Can you work these out from the model? Positions are in its coordinate system, mm. A direction names the side the tool comes from. Round coordinates to 2 decimals unless told otherwise and drop trailing zeros. One line per item, written item: value. Start each with the question number.
(1) I'm going to push flat-ended pins straight in: pin 1 Ø1.5 at (x, z) = (20, 6) entering from +Y; pin 2 Ø1 at (x, z) = (-0.5, 9.5) entering from +Y. Where does each tip first touch, or does it pass through?
(2) If I drill on L1, parallel to X at y = 33, z = 9.25; L2, parallel to X at y = 141.75, z = 6; L3, parallel to Z at x = 20, y = 140, over which ranges is the centre line in solid material (lowest first)? Write a range as from..to.
(3) Thinking about a two-plate mould opening in X: for faces 3 (the face through (72.5, -2, 5)), 4 (the face through (-1, 2, 0)), 5 (the face through (-42.44, 83.61, 9.68)), which applies, +X half, -X half, draft (parallel to the pull), parting line (faces both ways), or undercut?
(4) On a 3-axis mill with a long thin cutter (end or side, diameter ignored), from which of +Z, -Z, +X, -X, +Y, -Y can I reach the whole of each face in a straight line? I mean faces 1 (the face through (1, 145, 5)), 2 (the face through (43.94, 83.625, 9.679)). Say none if no direction works.
Autodesk Inventor part; units mm, degrees
ref_plane "YZ Plane" through (0, 0, 0) normal (1, 0, 0) x (0, 1, 0)
ref_plane "XZ Plane" through (0, 0, 0) normal (0, 1, 0) x (-1, 0, 0)
ref_plane "XY Plane" through (0, 0, 0) normal (0, 0, 1) x (1, 0, 0)
sketch "Sketch1" plane through (0, 0, 0) normal (0, 0, 1) x (1, 0, 0)
  line L0 (-72.5, -145) -> (72.5, -145)
  line L1 (72.5, -145) -> (72.5, 145)
  line L2 (72.5, 145) -> (-72.5, 145)
  line L3 (-72.5, 145) -> (-72.5, -145)
  line L4 (-72.5, -145) -> (72.5, 145) construction
  line L5 (72.5, -145) -> (-72.5, 145) construction
  point P0 (0, 0)
  dimension "d0" = 145
  dimension "d1" = 290
extrude "Extrusion1" add sketch "Sketch1" along normal blind 10
sketch "Sketch6" plane through (0, 0, 10) normal (0, 0, 1) x (1, 0, 0)
  line L0 (-72.5, -145) -> (72.5, -145)
  line L1 (72.5, -145) -> (72.5, 145)
  line L2 (72.5, 145) -> (-72.5, 145)
  line L3 (-72.5, 145) -> (-72.5, -145)
  arc A0 (-49.5, -81.8686) -> (49.5, -81.8686) centre (0, -81.8686) ccw
  line L4 (-49.5, 58.1314) -> (-49.5, -81.8686)
  line L5 (49.5, 58.1314) -> (49.5, -81.8686)
  line L6 (-72.5, 142) -> (72.5, 142)
  line L7 (72.5, -145) -> (72.5, 145)
  line L8 (-72.5, -145) -> (72.5, -145)
  line L9 (0, -145) -> (0, 145)
  line L10 (72.5, 145) -> (-72.5, 145)
  arc A1 (-24.5516, 102.6045) -> (-1.3, 142) centre (-46.3, 142) ccw
  arc A2 (1.3, 142) -> (24.5516, 102.6045) centre (46.3, 142) ccw
  line L11 (-50.8, -81.8686) -> (-50.8, 58.1314)
  line L12 (50.8, 58.1314) -> (50.8, -81.8686)
  arc A3 (-50.8, -81.8686) -> (50.8, -81.8686) centre (0, -81.8686) ccw
  arc A4 (-23.9233, 101.4664) -> (0, 142) centre (-46.3, 142) ccw
  arc A5 (0, 142) -> (23.9233, 101.4664) centre (46.3, 142) ccw
  arc A6 (50.8, 58.1314) -> (24.5516, 102.6045) centre (0, 58.1314) ccw
  arc A7 (-24.5516, 102.6045) -> (-50.8, 58.1314) centre (0, 58.1314) ccw
  arc A8 (49.5, 58.1314) -> (23.9233, 101.4664) centre (0, 58.1314) ccw
  arc A9 (-23.9233, 101.4664) -> (-49.5, 58.1314) centre (0, 58.1314) ccw
  point P0 (0, 0)
  dimension "d80" = 3
  dimension "d83" = 90
  dimension "d84" = 90
  dimension "d86" = 1.3
  dimension "d87" = 1.3
  dimension "d88" = 1.3
  dimension "d89" = 99
  dimension "d90" = 49.5
  dimension "d91" = 49.5
  dimension "d92" = 1.3
  dimension "d93" = 1.3
  dimension "d94" = 1.3
  dimension "d114" = 140
extrude "Extrusion12" cut sketch "Sketch6" against normal blind 1.3 contours A3 L11 A7 A1 L6 A4 A9 L4 A0 L9 | L9 A0 L5 A8 A5 L6 A2 A6 L12 A3
sketch "Sketch8" plane through (0, 0, 10) normal (0, 0, 1) x (1, 0, 0)
  line L0 (72.5, 145) -> (-72.5, 145)
  line L1 (72.5, -145) -> (72.5, 145)
  line L2 (-72.5, -145) -> (72.5, -145)
  line L3 (-72.5, 145) -> (-72.5, -145)
  line L4 (-1.3, 145) -> (1.3, 145)
  line L5 (1.3, 145) -> (1.3, 135)
  line L6 (1.3, 135) -> (-1.3, 135)
  line L7 (-1.3, 135) -> (-1.3, 145)
  point P0 (0, 0)
  dimension "d59" = 2.6
  dimension "d60" = 10
  dimension "d61" = 71.2
extrude "Extrusion10" cut sketch "Sketch8" against normal up to surface (1.3 mm away) contours L5 L6 L7 L0
sketch "Sketch9" plane through (-72.5, 145, 0) normal (0, 1, 0) x (1, 0, 0)
  line L0 (71.2, -8.7) -> (73.8, -8.7)
  line L1 (145, -10) -> (73.8, -10)
  line L2 (145, 0) -> (145, -10)
  line L3 (145, 0) -> (0, 0)
  line L4 (0, 0) -> (0, -10)
  line L5 (96.4233, -10) -> (73.0322, -10)
  line L6 (75.525, -10) -> (69.475, -10)
  line L7 (69.475, -10) -> (69.475, -5.67)
  line L8 (69.475, -5.67) -> (75.525, -5.67)
  line L9 (75.525, -5.67) -> (75.525, -10)
  line L10 (72.5, -5.67) -> (72.5, -10)
  line L11 (73.0322, -10) -> (71.9678, -10)
  line L12 (71.2, -10) -> (71.2, -8.7)
  line L13 (73.8, -8.7) -> (73.8, -10)
  line L14 (71.2, -10) -> (0, -10)
  point P0 (72.5, 0)
  point P1 (76.3, -7)
  dimension "d64" = 4.33
  dimension "d65" = 6.05
  dimension "d66" = 72.5
extrude "Extrusion14" [suppressed]
fillet "Fillet2" radius 0.65 14 edges at (-7.5464, 119.1273, 8.7) (-43.7485, 83.9521, 8.7) (-50.8, -11.8686, 8.7) (0, -132.6686, 8.7) (50.8, -11.8686, 8.7) (43.7485, 83.9521, 8.7) (7.5464, 119.1273, 8.7) (42.6289, 83.2913, 8.7) (49.5, -11.8686, 8.7) (0, -131.3686, 8.7) (-49.5, -11.8686, 8.7) (-42.6289, 83.2913, 8.7) (-8.3257, 115.5114, 8.7) (8.3257, 115.5114, 8.7)
sketch "Sketch12" plane through (-72.5, 145, 0) normal (0, 1, 0) x (1, 0, 0)
  line L0 (71.2, -10) -> (71.2, -9.35)
  arc A0 (71.85, -8.7) -> (71.2, -9.35) centre (71.85, -9.35) ccw
  line L1 (71.85, -8.7) -> (73.15, -8.7)
  arc A1 (73.8, -9.35) -> (73.15, -8.7) centre (73.15, -9.35) ccw
  line L2 (73.8, -9.35) -> (73.8, -10)
  line L3 (145, -10) -> (73.8, -10)
  line L4 (145, 0) -> (145, -10)
  line L5 (145, 0) -> (0, 0)
  line L6 (0, 0) -> (0, -10)
  line L7 (71.2, -10) -> (0, -10)
  line L8 (145, -10) -> (73.8, -10)
  line L9 (145, 0) -> (0, 0)
  line L10 (72.5, 0) -> (72.5, -6)
  line L11 (72.5, -6) -> (92.5, -6)
  line L12 (72.5, -6) -> (52.5, -6)
  dimension "d103" = 20
  dimension "d104" = 20
  dimension "d105" = 4
hole "Hole2" at (-20, 145, 6) at (20, 145, 6) direction (0, -1, 0) diameter 2.459 depth 8.8 tip angle 118
equation "\"d0\" = ScintillatorWidth"
equation "\"d1\" = ScintillatorHeight"
equation "\"d2\" = ScintillatorThickness"
equation "\"d80\" = ScintillatorEdgeClearence"
equation "\"d83\" = LoopSmallTrackDiameter"
equation "\"d84\" = LoopSmallTrackDiameter"
equation "\"d86\" = OpticalFiberDiameter + 2 * OpticalFiberClearence"
equation "\"d87\" = OpticalFiberDiameter + 2 * OpticalFiberClearence"
equation "\"d88\" = OpticalFiberDiameter + 2 * OpticalFiberClearence"
equation "\"d92\" = OpticalFiberDiameter + 2 * OpticalFiberClearence"
equation "\"d93\" = OpticalFiberDiameter + 2 * OpticalFiberClearence"
equation "\"d94\" = OpticalFiberDiameter + 2 * OpticalFiberClearence"
equation "\"d95\" = OpticalFiberDiameter + 2 * OpticalFiberClearence"
equation "\"d59\" = 4 * OpticalFiberClearence + 2 * OpticalFiberDiameter"
equation "\"d61\" = 0.5 * ScintillatorWidth - 2 * OpticalFiberClearence - OpticalFiberDiameter"
equation "\"d62\" = ShallowTrackDepth"
equation "\"d65\" = MPPCWidth + 2 * MPPCClearence"
equation "\"d66\" = 0.5 * ScintillatorWidth"
equation "\"d99\" = MPPCDepth"
equation "\"d5\" = OpticalFiberDiameter + 2 * OpticalFiberClearence"
equation "\"d21\" = d5"
equation "\"d22\" = d5"
equation "\"OpticalFiberDiameter\" = 1"
equation "\"ScintillatorThickness\" = 10"
equation "\"OpticalFiberClearence\" = 0.15"
equation "\"SmallTrackDiameter\" = 175"
equation "\"ScintillatorEdgeClearence\" = 3"
equation "\"ScintillatorWidth\" = 145"
equation "\"ScintillatorHeight\" = 290"
equation "\"ShallowTrackDepth\" = 1.3"
equation "\"MPPCClearence\" = 0.075"
equation "\"MPPCSensorClearence\" = 1.45"
equation "\"MPPCSensorOffsett\" = 2.105"
equation "\"MPPCWidth\" = 5.9"
equation "\"MPPCHeight\" = 6.55"
equation "\"FiberEdgeOffsett\" = 5"
equation "\"MPPCDepth\" = 1"
equation "\"LongFiberAngle\" = 30deg"
equation "\"ShortFiberAngle\" = 78deg"
equation "\"LoopLargeTrackRatio\" = 1.1"
equation "\"LoopSmallTrackDiameter\" = 90"
equation "\"FiberSensorClerence\" = 0.5"
equation "\"MountingScrewDepth\" = 4"
properties part number "Scintillator Tile" material "ABS Plastic"
Established:
1. pin 1: y = 135.91
1. pin 2: y = 135
2. L1: -72.5..-50.79, -49.51..49.51, 50.79..72.5
2. L2: -72.5..-21.23, -18.77..18.77, 21.23..72.5
2. L3: 0..4.77, 7.23..10
3. face 3: +X half
3. face 4: draft
3. face 5: undercut
4. face 1: +Z, -Z, +X, -X, +Y
4. face 2: +Z
